Here's how the part is built. I have some questions about the finished solid (model axes, mm). Face numbers are marked on the shaded views. A direction names the side the tool comes from. Round coordinates to 2 decimals unless told otherwise and drop trailing zeros. Loops run counter-clockwise (first coordinate to the right, second up) from the corner with the lowest first, then second, coordinate; pieces in that order, holes last. Notation, with made-up numbers: M 66,-20.75 L 92,-20.75 A22 ccw 92,2.25 Z; hole C 17.25,-15.75 d1. An arc over 180 degrees is marked long. Answer as a JSON object with one key per item and string values.
from build123d import *

# Parameters (mm, degrees)
F0_R      = 4.1669678751
F2_DEPTH  = 1.27
F3_R      = 3.429
F4_DEPTH  = 0.762
F5_W      = 5.5987872183
F5_H      = 6.2324469909
F6_DEPTH  = 0.508
F7_R      = 4.1275
F8_DEPTH  = 1.016
F10_W     = 0.2829879522
F10_H     = 0.2722851932
F11_DEPTH = 3.2766
F14_R     = 0.4905681959
F15_R     = 0.4292471714
F16_R     = 0.1839630735


with BuildPart() as f2:
    # F0 (on Top) → F2 (new body)
    with BuildSketch(Plane.XY):
        with Locations((-38.0157418549, 10.2490512654)):
            Circle(F0_R)
    extrude(amount=F2_DEPTH)

    # F3 (on face) → F4 (join)
    with BuildSketch(Plane.XY.offset(1.27)):
        with Locations((-38.0157418549, 10.2490512654)):
            Circle(F3_R)
    extrude(amount=F4_DEPTH)

    # F5 (on face) → F6 (join)
    with BuildSketch(Plane.XY.offset(2.032)):
        with Locations((-37.9977691919, 10.2676521055)):
            Rectangle(F5_W, F5_H)
    extrude(amount=F6_DEPTH)

    # F7 (on face) → F8 (join)
    with BuildSketch(Plane.XY.offset(2.54)):
        with Locations((-37.9977691919, 10.2307982743)):
            Circle(F7_R)
    extrude(amount=F8_DEPTH)

    # F10 (on face) → F11 (join)
    with BuildSketch(Plane.XY.offset(3.556)):
        with Locations((-38.0135253072, 10.2514149621)):
            Rectangle(F10_W, F10_H)
    extrude(amount=F11_DEPTH)

    # F12 (on face) → F13 (revolve)
    with BuildSketch(Plane(origin=(-38.1550192833, 0, 0), x_dir=(0, -1, 0), z_dir=(-1, 0, 0))):
        with BuildLine():
            Line((-10.3875575587, 5.6081162018), (-10.3875575587, 6.7985399348))
            ThreePointArc((-10.3875575587, 6.7985399348), (-10.8013159849, 6.2033280683), (-10.3875575587, 5.6081162018))
        make_face()
    revolve(axis=Axis((-38.1550192833, 10.1152723655, 5.1943), (0, 0, -1)))

    # F14
    f14_edges = [f2.edges().sort_by_distance(p)[0] for p in [
        (-42.125269, 10.230798, 3.556),
        (-37.872031, 10.251415, 3.556),
        (-38.013525, 10.387558, 3.556),
        (-38.155019, 10.251415, 3.556),
        (-38.013525, 10.115272, 3.556),
    ]]
    fillet(f14_edges, radius=F14_R)

    # F15
    f15_edges = [f2.edges().sort_by_distance(p)[0] for p in [
        (-42.18271, 10.249051, 0),
    ]]
    fillet(f15_edges, radius=F15_R)

    # F16
    f16_edges = [f2.edges().sort_by_distance(p)[0] for p in [
        (-42.18271, 10.249051, 1.27),
    ]]
    fillet(f16_edges, radius=F16_R)


solid = f2.part
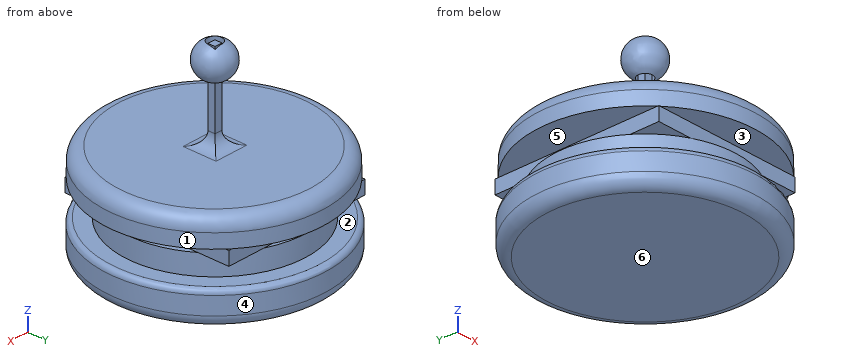
Item 1: If we mould it in two halves opening along Z, with no side actions, what happens to the marked faces 4, 5 and 6? For each: pulls with the +Z half, pulls with the -Z half, needs draft (parallel to the pull), parting line crosses it, or undercut.
Resolved:
{"face 4": "needs draft", "face 5": "undercut", "face 6": "pulls with the -Z half"}
Item 2: I'm going to push flat-ended pins straight in: pin 1 Ø2.5 at (x, y) = (-38.5, 9.5) entering from +Z; pin 2 Ø0.6 at (y, z) = (11, 2.5) entering from -X; pin 3 Ø4 at (y, z) = (12, 4.5) entering from +X; pin 4 Ø1 at (y, z) = (9, 2) entering from +X. Where does each tip first touch, or does it pass through?
Resolved:
{"pin 1": "z = 6.83", "pin 2": "x = -42.1", "pin 3": "x = -33.89", "pin 4": "x = -34.67"}
Item 3: On a 3-axis mill with a long thin cutter (end or side, diameter ignored), from which of +Z, -Z, +X, -X, +Y, -Y can I reach the whole of each face in a straight line? I mean the marked faces 1, 2 and 3. Say none if no direction works.
Resolved:
{"face 1": "+Z", "face 2": "none", "face 3": "+X, -X, -Y"}
Item 4: I want a section at A-A, the plane z = 5. Please give me the cut outline in (x, y), then the cut area to 3 significant figures.
Resolved:
{"outline": "M -38.16,10.12 L -37.87,10.12 L -37.87,10.39 L -38.16,10.39 Z", "area": "0.0771 mm²"}
Item 5: I want a section at B-B, the plane z = 0.75. Please give me the cut outline in (x, y).
Resolved:
{"outline": "C -38.02,10.25 d8.33"}
Item 6: Please list where these lines run through material, in increasing order: probe 1 along Z at (x, y) = (-37.5, 12.5); probe 2 along X at (y, z) = (10.25, 2.5); probe 3 along Z at (x, y) = (-38.75, 10). Write a range as from..to.
Resolved:
{"probe 1": "0..3.56", "probe 2": "-40.8..-35.2", "probe 3": "0..3.56, 5.89..6.51"}
